The listing builds one solid part. Answer for the finished solid, in the listing's coordinates (mm). Round coordinates to 2 decimals unless told otherwise and drop trailing zeros. Write each loop counter-clockwise with the first axis right and the second up, starting at its lowest first coordinate (ties: lowest second). Pieces come first, ordered by that corner, then holes.
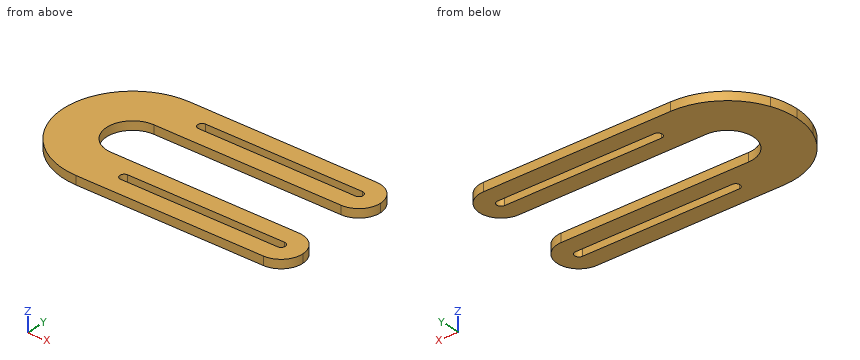
Autodesk Inventor part; units mm, degrees
ref_plane "YZ Plane" through (0, 0, 0) normal (1, 0, 0) x (0, 1, 0)
ref_plane "XZ Plane" through (0, 0, 0) normal (0, 1, 0) x (-1, 0, 0)
ref_plane "XY Plane" through (0, 0, 0) normal (0, 0, 1) x (1, 0, 0)
sketch "Sketch1" plane through (0, 0, 0) normal (0, 0, 1) x (1, 0, 0)
  line L0 (0, 0) -> (162.56, 0)
  line L1 (162.56, 0) -> (162.56, 81.28)
  line L2 (162.56, 81.28) -> (0, 81.28)
  line L3 (0, 81.28) -> (0, 0)
  dimension "d0" = 162.56
  dimension "d1" = 81.28
extrude "Extrusion1" add sketch "Sketch1" along normal blind 5.08
sketch "Sketch2" plane through (0, 0, 5.08) normal (0, 0, 1) x (1, 0, 0)
  line L0 (0, 0) -> (162.56, 0)
  line L1 (162.56, 0) -> (162.56, 81.28)
  line L2 (162.56, 81.28) -> (0, 81.28)
  line L3 (0, 81.28) -> (0, 0) construction
  line L4 (0, 40.64) -> (162.56, 40.64) construction
  arc A0 (40.64, 55.88) -> (40.64, 25.4) centre (40.64, 40.64) ccw
  arc A1 (78.3143, 55.88) -> (40.64, 81.28) centre (40.64, 40.64) ccw construction
  line L5 (0, 81.28) -> (0, 0)
  line L6 (0, 0) -> (162.56, 0)
  line L7 (0, 81.28) -> (40.64, 81.28) construction
  line L8 (162.56, 81.28) -> (162.56, 0)
  line L9 (162.56, 0) -> (40.64, 0)
  line L10 (0, 0) -> (0, 40.64)
  line L11 (0, 40.64) -> (0, 81.28)
  line L12 (40.64, 0) -> (0, 0) construction
  line L13 (40.64, 81.28) -> (162.56, 81.28)
  line L14 (40.64, 25.4) -> (78.3143, 25.4)
  line L15 (40.64, 55.88) -> (78.3143, 55.88)
  line L16 (162.56, 0) -> (162.56, 81.28)
  line L17 (162.56, 23.2866) -> (162.56, 55.88)
  line L18 (40.64, 25.4) -> (78.3143, 25.4)
  line L19 (162.56, 25.4) -> (162.56, 55.88) construction
  line L20 (162.56, 55.88) -> (40.64, 55.88)
  line L21 (40.64, 55.88) -> (40.64, 25.4) construction
  arc A2 (55.88, 40.64) -> (40.64, 55.88) centre (40.64, 40.64) ccw construction
  arc A3 (40.64, 25.4) -> (55.88, 40.64) centre (40.64, 40.64) ccw construction
  arc A4 (81.28, 40.64) -> (78.3143, 55.88) centre (40.64, 40.64) ccw construction
  arc A5 (78.3143, 25.4) -> (81.28, 40.64) centre (40.64, 40.64) ccw construction
  arc A6 (40.64, 81.28) -> (2.9657, 55.88) centre (40.64, 40.64) ccw
  arc A7 (40.64, 0) -> (78.3143, 25.4) centre (40.64, 40.64) ccw construction
  arc A8 (0, 40.64) -> (2.9657, 25.4) centre (40.64, 40.64) ccw
  arc A9 (2.9657, 25.4) -> (40.64, 0) centre (40.64, 40.64) ccw
  arc A10 (2.9657, 55.88) -> (0, 40.64) centre (40.64, 40.64) ccw
  line L22 (78.3143, 55.88) -> (162.56, 55.88)
  line L23 (78.3143, 25.4) -> (162.56, 25.4)
  line L24 (78.3143, 25.4) -> (162.56, 25.4)
  dimension "d4" = 30.48
extrude "Extrusion2" cut sketch "Sketch2" against normal blind 5.08 contours A9 A8 A10 A6 L2 L1 L20 L15 A0 L14 L23 L0 keep common part
sketch "Sketch3" plane through (0, 0, 5.08) normal (0, 0, 1) x (1, 0, 0)
  line L0 (162.56, 55.88) -> (40.64, 55.88)
  line L1 (162.56, 55.88) -> (162.56, 81.28)
  line L2 (162.56, 81.28) -> (40.64, 81.28)
  arc A0 (40.64, 81.28) -> (40.64, 0) centre (40.64, 40.64) ccw
  line L3 (40.64, 0) -> (162.56, 0)
  line L4 (162.56, 0) -> (162.56, 25.4)
  line L5 (40.64, 25.4) -> (162.56, 25.4)
  arc A1 (40.64, 55.88) -> (40.64, 25.4) centre (40.64, 40.64) ccw
  line L6 (40.64, 40.64) -> (162.56, 40.64) construction
  line L7 (162.56, 40.64) -> (162.56, 25.4) construction
  line L8 (58.42, 68.58) -> (149.86, 68.58) construction
  line L9 (58.42, 66.08) -> (149.86, 66.08)
  line L10 (149.86, 71.08) -> (58.42, 71.08)
  arc A2 (58.42, 71.08) -> (58.42, 66.08) centre (58.42, 68.58) ccw
  arc A3 (149.86, 66.08) -> (149.86, 71.08) centre (149.86, 68.58) ccw
  line L11 (40.64, 55.88) -> (40.64, 81.28) construction
  line L12 (58.42, 12.7) -> (149.86, 12.7) construction
  line L13 (58.42, 15.2) -> (149.86, 15.2)
  line L14 (149.86, 10.2) -> (58.42, 10.2)
  arc A4 (58.42, 15.2) -> (58.42, 10.2) centre (58.42, 12.7) ccw
  arc A5 (149.86, 10.2) -> (149.86, 15.2) centre (149.86, 12.7) ccw
  point P0 (0, 0)
  point P1 (104.14, 68.58)
  point P2 (104.14, 12.7)
  dimension "d7" = 2.5
  dimension "d8" = 121.92
  dimension "d10" = 25.4
  dimension "d11" = 12.7
  dimension "d12" = 91.44
  dimension "d13" = 12.7
extrude "Extrusion3" cut sketch "Sketch3" against normal blind 5.08 contours A2 L10 A3 L9 | L13 A5 L14 A4
fillet "Fillet1" radius 12.7 4 edges at (162.56, 0, 2.54) (162.56, 25.4, 2.54) (162.56, 55.88, 2.54) (162.56, 81.28, 2.54)
equation "\"d0\" = 2 * d1"
equation "\"d11\" = 0.5 * d10"
equation "\"d13\" = d11"
properties part number "SuctionGrabberA" material "Wood (Birch)"
1. Given pin 1 (1 mm diameter, centred on x = 81.5, y = 54.5, fed in from +Z); pin 2 (2 mm diameter, centred on y = 72.5, z = 4.5, fed in from +X), each flat-ended and moving along its own axis, determine where each tip first touches the part or whether it passes through.
Geometry says:
pin 1: passes through
pin 2: stops at x = 162.22
2. Section D-D on x = 22.5 is taken. Determine the outline of the cut face in (y, z).
Geometry says:
outline: (4.27, 0) - (77.01, 0) - (77.01, 5.08) - (4.27, 5.08) - close
3. Straight lines are drawn through the part: line 1 along Y through (x, z) = (144, 0.65); line 2 along Y through (x, z) = (30.5, 3.05); line 3 along X through (y, z) = (12.5, 0.55). For each, find the intervals that lie inside material, in ascending order.
Geometry says:
line 1: y = 0 to 10.2, 15.2 to 25.4, 55.88 to 66.08, 71.08 to 81.28
line 2: y = 1.29 to 29.26, 52.02 to 79.99
line 3: x = 11.32 to 55.93, 152.35 to 162.56
4. Section A-A on z = 2.7 is taken. Give the number of separate pieces and of enclosed holes in the cut face, plus the area to 3 significant figures.
Geometry says:
separate pieces: 1
enclosed holes: 2
area: 7,330 mm2
5. Section B-B on x = 93.5 is taken. Determine the outline of the cut face in (y, z).
Geometry says:
outline: (0, 0) - (10.2, 0) - (10.2, 5.08) - (0, 5.08) - close; (15.2, 0) - (25.4, 0) - (25.4, 5.08) - (15.2, 5.08) - close; (55.88, 0) - (66.08, 0) - (66.08, 5.08) - (55.88, 5.08) - close; (71.08, 0) - (81.28, 0) - (81.28, 5.08) - (71.08, 5.08) - close
6. Section C-C on y = 32 is taken. Determine the outline of the cut face in (x, z), plus the area to 3 significant figures.
Geometry says:
outline: (0.93, 0) - (28.09, 0) - (28.09, 5.08) - (0.93, 5.08) - close
area: 138 mm2
